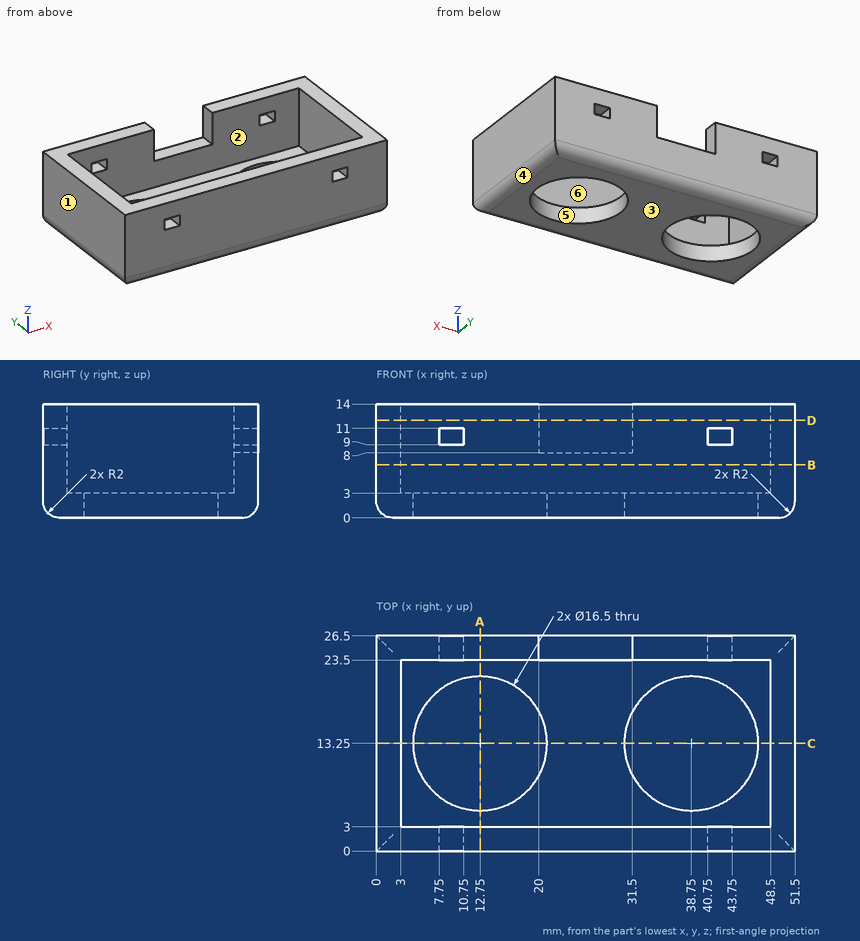
Print and shaded views of the part. All mm, measured from the part's lowest x, y and z. A direction names the side the tool comes from. Round coordinates to 2 decimals unless told otherwise and drop trailing zeros. Write each loop counter-clockwise with the first axis right and the second up, starting at its lowest first coordinate (ties: lowest second). Pieces come first, ordered by that corner, then holes.
Item 1: Cut at A-A, the plane x = 12.75. Give the cut face in (y, z).
Results:
outline: (0, 2) arc R2 ccw to (2, 0) - (5, 0) - (5, 3) - (3, 3) - (3, 14) - (0, 14) - close; (21.5, 0) - (24.5, 0) arc R2 ccw to (26.5, 2) - (26.5, 14) - (23.5, 14) - (23.5, 3) - (21.5, 3) - close
Item 2: Probe L1, parallel to Y at x = 39.5, z = 7.25; L2, parallel to Y at x = 38.75, z = 2.3; L3, parallel to X at y = 17.5, z = 10.5. List the from-to ranges inside material, lowest first.
Results:
L1: y = 0 to 3, 23.5 to 26.5
L2: y = 0 to 5, 21.5 to 26.5
L3: x = 0 to 3, 48.5 to 51.5
Item 3: Which spindle directions (+Z, -Z, +X, -X, +Y, -Y) get a long thin tool onto all of the face, cutting with end or side? Do the marked faces 5 and 6. Say none if no direction does.
Results:
face 5: +Z, -Z
face 6: +Z
Item 4: Cut at D-D, the plane z = 12. Give the cut face in (x, y), plus the area to 4 significant figures.
Results:
outline: (0, 0) - (51.5, 0) - (51.5, 26.5) - (31.5, 26.5) - (31.5, 23.5) - (48.5, 23.5) - (48.5, 3) - (3, 3) - (3, 23.5) - (20, 23.5) - (20, 26.5) - (0, 26.5) - close
area: 397.5 mm2
Item 5: Two-plate mould, pull along X, no slides. Class the marked faces 1, 2, 3 and 4: +X half, -X half, draft (parallel to the pull), parting line (faces both ways), or undercut.
Results:
face 1: -X half
face 2: undercut
face 3: draft
face 4: +X half
Item 6: Cut at C-C, the plane y = 13.25. Give the cut face in (x, z).
Results:
outline: (0, 2) arc R2 ccw to (2, 0) - (4.5, 0) - (4.5, 3) - (3, 3) - (3, 14) - (0, 14) - close; (21, 0) - (30.5, 0) - (30.5, 3) - (21, 3) - close; (47, 0) - (49.5, 0) arc R2 ccw to (51.5, 2) - (51.5, 14) - (48.5, 14) - (48.5, 3) - (47, 3) - close
Item 7: Drop flat-ended pins along their axis: pin 1 Ø4 at (x, y) = (10, 9) entering from -Z; pin 2 Ø8 at (x, y) = (43.5, 13) entering from +Z; pin 3 Ø2.5 at (x, y) = (28, 24.5) entering from +Z. Give the stop position or say it passes through.
Results:
pin 1: passes through
pin 2: stops at z = 3
pin 3: stops at z = 8
Item 8: Cut at B-B, the plane z = 6.5. Give the cut face in (x, y), plus the area to 3 significant figures.
Results:
outline: (0, 0) - (51.5, 0) - (51.5, 26.5) - (0, 26.5) - close; hole (3, 3) - (48.5, 3) - (48.5, 23.5) - (3, 23.5) - close
area: 432 mm2
